CAD build for the part. Positions are in the model's coordinates, mm. Coordinates: 2 decimals unless noted, no trailing zeros. Order: outer loops, then holes, each group sorted by start corner. A loop starts at its lowest first (then second) coordinate and runs counter-clockwise, first axis right, second up. Notation, with made-up numbers: (24, 74.5) - (75, 74.5) arc R30 ccw to (75, 108.5) - close; hole circle Ø2 at (58, 84.25). An arc over 180 degrees is marked (long way). Use one line per item in the form item = value.
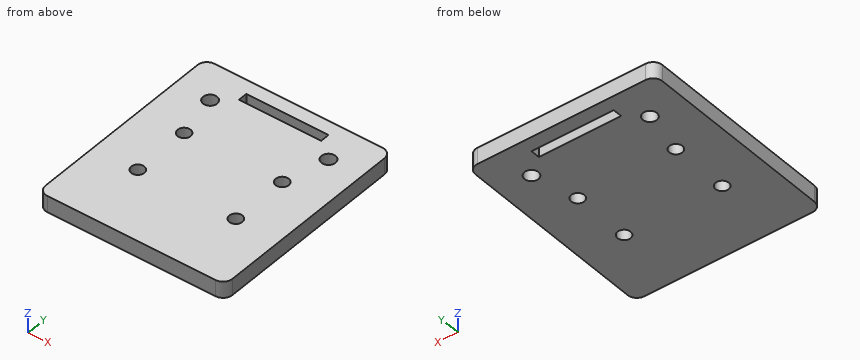
```python
from build123d import *

# Parameters (mm, degrees)
BOSS_EXTRUDE1_DEPTH = 3.5
SKETCH2_W           = 8.8
SKETCH2_H           = 2
CUT_EXTRUDE1_DEPTH  = 61.309617744
SKETCH3_R           = 1.5
CUT_EXTRUDE2_DEPTH  = 61.309617744
SKETCH4_R           = 1.4
CUT_EXTRUDE3_DEPTH  = 61.309617744


with BuildPart() as part:
    # Sketch1 → Boss-Extrude1 (new body)
    with BuildSketch(Plane.XY):
        with BuildLine():
            Line((-2, 0), (-38, 0))
            ThreePointArc((-38, 0), (-39.414213562, 0.585786438), (-40, 2))
            Line((-40, 2), (-40, 42.999999916))
            ThreePointArc((-40, 42.999999916), (-39.414213562, 44.414213478), (-38, 44.999999916))
            Line((-38, 44.999999916), (-2, 44.999999916))
            ThreePointArc((-2, 44.999999916), (-0.585786438, 44.414213478), (0, 42.999999916))
            Line((0, 42.999999916), (0, 2))
            ThreePointArc((0, 2), (-0.585786438, 0.585786438), (-2, 0))
        make_face()
    extrude(amount=BOSS_EXTRUDE1_DEPTH)

    # Sketch2 → Cut-Extrude1 (cut, through all)
    with BuildSketch(Plane.XY.offset(3.5)):
        with Locations((-24.4, 41.033946817)):
            Rectangle(SKETCH2_W, SKETCH2_H)
        with Locations((-15.6, 41.033946817)):
            Rectangle(SKETCH2_W, SKETCH2_H)
    extrude(amount=-CUT_EXTRUDE1_DEPTH, mode=Mode.SUBTRACT)

    # Sketch3 → Cut-Extrude2 (cut, through all)
    with BuildSketch(Plane.XY.offset(3.5)):
        with Locations((-32.512621431, 36.953417216)):
            Circle(SKETCH3_R)
        with Locations((-7.172621431, 36.953417216)):
            Circle(SKETCH3_R)
    extrude(amount=-CUT_EXTRUDE2_DEPTH, mode=Mode.SUBTRACT)

    # Sketch4 → Cut-Extrude3 (cut, through all)
    with BuildSketch(Plane.XY.offset(3.5)):
        with Locations((-30.5, 27.406241852)):
            Circle(SKETCH4_R)
        with Locations((-30.5, 14.906241852)):
            Circle(SKETCH4_R)
        with Locations((-9.5, 14.906241852)):
            Circle(SKETCH4_R)
        with Locations((-9.5, 27.406241852)):
            Circle(SKETCH4_R)
    extrude(amount=-CUT_EXTRUDE3_DEPTH, mode=Mode.SUBTRACT)


solid = part.part
```
Item 1: Cut at A-A, the plane x = -9.5. Write the cut outline in (y, z).
Derived:
outline = (0, 0) - (13.51, 0) - (13.51, 3.5) - (0, 3.5) - close; (16.31, 0) - (26.01, 0) - (26.01, 3.5) - (16.31, 3.5) - close; (28.81, 0) - (45, 0) - (45, 3.5) - (28.81, 3.5) - close
Item 2: Cut at B-B, the plane x = -28. Write the cut outline in (y, z), plus the area to 4 significant figures.
Derived:
outline = (0, 0) - (40.03, 0) - (40.03, 3.5) - (0, 3.5) - close; (42.03, 0) - (45, 0) - (45, 3.5) - (42.03, 3.5) - close
area = 150.5 mm²
Item 3: Cut at C-C, the plane z = 0.7. Write the cut outline in (x, y), plus the area to 3 significant figures.
Derived:
outline = (-40, 2) arc R2 ccw to (-38, 0) - (-2, 0) arc R2 ccw to (0, 2) - (0, 43) arc R2 ccw to (-2, 45) - (-38, 45) arc R2 ccw to (-40, 43) - close; hole circle Ø3 at (-32.51, 36.95); hole circle Ø2.8 at (-30.5, 14.91); hole circle Ø2.8 at (-30.5, 27.41); hole (-28.8, 40.03) - (-11.2, 40.03) - (-11.2, 42.03) - (-28.8, 42.03) - close; hole circle Ø2.8 at (-9.5, 14.91); hole circle Ø2.8 at (-9.5, 27.41); hole circle Ø3 at (-7.17, 36.95)
area = 1,720 mm²
Item 4: Drill centre lines: line 1 (X direction, y = 15, z = 3.2); line 2 (Y direction, x = -12.5, z = 0.6); line 3 (Y direction, x = -6, z = 0.65). Where is each one in solid material? Low to high. Write a range as [from, to].
Derived:
line_1 = [-40, -31.9], [-29.1, -10.9], [-8.1, 0]
line_2 = [0, 40.03], [42.03, 45]
line_3 = [0, 36.02], [37.89, 45]
